from build123d import *

# Parameters (mm, degrees)
F0_W     = 21.844
F0_H     = 13.462
F1_DEPTH = 9.652
F3_D     = 2.8194
F5_DEPTH = 13.463


with BuildPart() as f1:
    # F0 (on Front) → F1 (new body)
    with BuildSketch(Plane.XZ):
        Rectangle(F0_W, F0_H)
    extrude(amount=F1_DEPTH)

    # F3 (through all)
    with Locations(Plane.XZ.offset(9.652)):
        with Locations((-7.1374, 0), (7.1374, 0)):
            Hole(F3_D / 2)

    # F4 (on face) → F5 (cut, through all)
    with BuildSketch(Plane.XY.offset(6.731)):
        with BuildLine():
            ThreePointArc((-4.7625, 0), (0, -4.7625), (4.7625, 0))
            Line((4.7625, 0), (-4.7625, 0))
        make_face()
    extrude(amount=-F5_DEPTH, mode=Mode.SUBTRACT)


solid = f1.part
CAD build for the part. Positions are in the model's coordinates, mm. Give positions to 0.01 mm unless a question says otherwise; leave off trailing zeros. Write each loop counter-clockwise with the first axis right and the second up, starting at its lowest first coordinate (ties: lowest second). Pieces come first, ordered by that corner, then holes. Notation, with made-up numbers: (87, 54.5) - (104, 54.5) arc R30 cw to (104, 80.5) - close; hole circle Ø2 at (58, 33.25). An arc over 180 degrees is marked (long way). Put each result on its own line as item: value.
(1) Saw through at D-D (x = -6.25). List the corners of the cut face in (y, z).
Working result:
outline: (-9.65, -6.73) - (0, -6.73) - (0, -1.1) - (-9.65, -1.1) - close; (-9.65, 1.1) - (0, 1.1) - (0, 6.73) - (-9.65, 6.73) - close
(2) Saw through at B-B (z = 0). List the corners of the cut face in (x, y) (1 decimal), then the cut area to 3 significant figures.
Working result:
outline: (-10.9, -9.7) - (-8.5, -9.7) - (-8.5, 0) - (-10.9, 0) - close; (-5.7, -9.7) - (5.7, -9.7) - (5.7, 0) - (4.8, 0) arc R4.8 cw to (-4.8, 0) - (-5.7, 0) - close; (8.5, -9.7) - (10.9, -9.7) - (10.9, 0) - (8.5, 0) - close
area: 121 mm^2
(3) Wall check: L1, parallel to X at y = -5.75, z = 0.5; L2, parallel to X at y = -1, z = 1; L3, parallel to Y at x = 0, z = -4.75. Give the ranges that are in metal, low to high.
Working result:
L1: -10.92 to -8.46, -5.82 to 5.82, 8.46 to 10.92
L2: -10.92 to -8.13, -6.14 to -4.66, 4.66 to 6.14, 8.13 to 10.92
L3: -9.65 to -4.76
(4) Saw through at C-C (y = -8.75). List the corners of the cut face in (x, z), then the cut area to 3 significant figures.
Working result:
outline: (-10.92, -6.73) - (10.92, -6.73) - (10.92, 6.73) - (-10.92, 6.73) - close; hole circle Ø2.82 at (-7.14, 0); hole circle Ø2.82 at (7.14, 0)
area: 282 mm^2
(5) Saw through at A-A (y = -1.25). List the corners of the cut face in (x, z).
Working result:
outline: (-10.92, -6.73) - (-4.6, -6.73) - (-4.6, 6.73) - (-10.92, 6.73) - close; (4.6, -6.73) - (10.92, -6.73) - (10.92, 6.73) - (4.6, 6.73) - close; hole circle Ø2.82 at (-7.14, 0); hole circle Ø2.82 at (7.14, 0)
(6) Pull direction Z, two halves, no side cores. Call faces 1 (the cylindrical face through (-8.482, -4.758, 0.423)), 2 (the flat face through (9, 0, 0)), 3 (the flat face through (0, -6, -6.731)): released by +Z, released by -Z, zero draft, split by the parting line, or undercut.
Working result:
face 1: undercut
face 2: zero draft
face 3: released by -Z
